from build123d import *

# Parameters (mm, degrees)
BASE_EXTRUDE_DEPTH = 12.7
LPATTERN1_COUNT    = 2
LPATTERN1_PITCH    = 20.6375


with BuildPart() as part:
    # Sketch1 → Base-Extrude (new, symmetric)
    with BuildSketch(Plane.XY):
        with BuildLine():
            Line((-20.6375, 9.37895), (-20.6375, -7.874))
            ThreePointArc((-20.6375, -7.874), (-20.33992049, -8.59242049), (-19.6215, -8.89))
            Line((-19.6215, -8.89), (-1.016, -8.89))
            ThreePointArc((-1.016, -8.89), (-0.29757951, -8.59242049), (0, -7.874))
            Line((0, -7.874), (0, 9.37895))
            ThreePointArc((0, 9.37895), (-2.38125, 11.7602), (-4.7625, 9.37895))
            Line((-4.7625, 9.37895), (-3.7465, 9.37895))
            ThreePointArc((-3.7465, 9.37895), (-2.38125, 10.7442), (-1.016, 9.37895))
            Line((-1.016, 9.37895), (-1.016, -7.874))
            Line((-1.016, -7.874), (-19.6215, -7.874))
            Line((-19.6215, -7.874), (-19.6215, 9.37895))
            ThreePointArc((-19.6215, 9.37895), (-18.25625, 10.7442), (-16.891, 9.37895))
            Line((-16.891, 9.37895), (-15.875, 9.37895))
            ThreePointArc((-15.875, 9.37895), (-18.25625, 11.7602), (-20.6375, 9.37895))
        make_face()
    base_extrude = extrude(amount=BASE_EXTRUDE_DEPTH, both=True)

    # LPattern1: Base-Extrude ×2
    with Locations(*[(i * LPATTERN1_PITCH, 0, 0) for i in range(1, LPATTERN1_COUNT)]):
        add(base_extrude)


solid = part.part
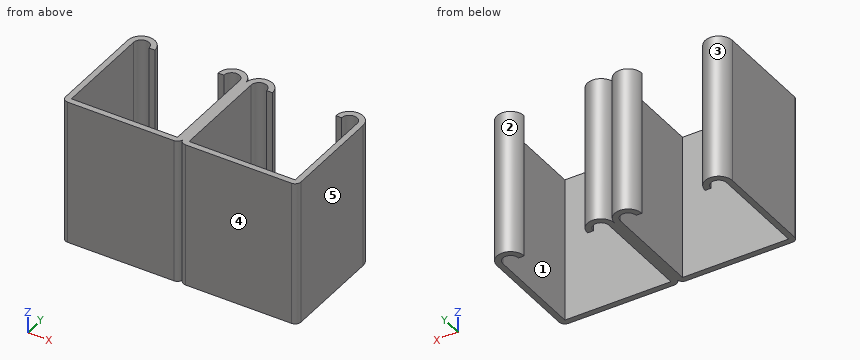
Read the model definition and answer for the solid it produces. Units are mm, in the model's axes. Face numbers are marked on the shaded views. A direction names the side the tool comes from. Give positions to 0.01 mm unless a question says otherwise; leave off trailing zeros. Write each loop counter-clockwise with the first axis right and the second up, starting at its lowest first coordinate (ties: lowest second). Pieces come first, ordered by that corner, then holes. Notation, with made-up numbers: (-37, 23.5) - (1, 23.5) arc R9 ccw to (1, 33.5) - close; hole circle Ø6 at (83.5, 81.5). An arc over 180 degrees is marked (long way). Use CSV: the item, a comma, the result in double quotes. Start each with the question number.
Item 1: The part is cut by section D-D, the plane x = 14. Give the vertices of the cut face in (y, z), and give its area (3 significant figures).
Item 2: The part is cut by section A-A, the plane y = 6.25. Give the vertices of the cut face in (x, z).
Item 3: The mould has two halves that part along X. Classify the marked faces 3, 4 and 5: pulls with the +X half, pulls with the -X half, needs draft (parallel to the pull), parting line crosses it, or undercut.
Item 4: The part is cut by section B-B, the plane x = -1.5. Give the vertices of the cut face in (y, z).
Item 5: Flat-ended cylindrical pins translate along their axes: P1, Ø5, axis at x = -9, y = 9.5, coming from the -Z side; P2, Ø9.5, axis at x = -9, z = -2, coming from the +Y side. Find the tip coordinate at first contact, or state that the pin passes through.
Item 6: Consider line 1 (X direction, y = 4.5, z = 5); line 2 (Y direction, x = -10, z = -3.5); line 3 (Y direction, x = 18.5, z = 9.75). Determine where each line is inside the solid, lowest interval first.
Item 7: The part is cut by section C-C, the plane z = -1.5. Give the vertices of the cut face in (x, y) (1 decimal), and give its area (3 significant figures).
Item 8: For the marked faces 1 and 2, determine the directions among +Z, -Z, +X, -X, +Y, -Y from which every point of the face is accessible in a straight line to the end or side of a thin tool.
Taken from the geometry:
1,outline,"(-8.89, -12.7) - (-7.87, -12.7) - (-7.87, 12.7) - (-8.89, 12.7) - close"
1,area,"25.8 mm2"
2,outline,"(-20.64, -12.7) - (-19.62, -12.7) - (-19.62, 12.7) - (-20.64, 12.7) - close; (-1.02, -12.7) - (1.02, -12.7) - (1.02, 12.7) - (-1.02, 12.7) - close; (19.62, -12.7) - (20.64, -12.7) - (20.64, 12.7) - (19.62, 12.7) - close"
3,face 3,"undercut"
3,face 4,"needs draft"
3,face 5,"pulls with the +X half"
4,outline,"(-8.89, -12.7) - (-7.87, -12.7) - (-7.87, 12.7) - (-8.89, 12.7) - close; (10.42, -12.7) - (11.59, -12.7) - (11.59, 12.7) - (10.42, 12.7) - close"
5,P1,"through"
5,P2,"y = 10.85"
6,line 1,"-20.64 to -19.62, -1.02 to 1.02, 19.62 to 20.64"
6,line 2,"-8.89 to -7.87"
6,line 3,"-8.89 to -7.87, 10.72 to 11.75"
7,outline,"(-20.6, -7.9) arc R1 ccw to (-19.6, -8.9) - (-1, -8.9) arc R1 ccw to (0, -7.9) arc R1 ccw to (1, -8.9) - (19.6, -8.9) arc R1 ccw to (20.6, -7.9) - (20.6, 9.4) arc R2.4 ccw to (15.9, 9.4) - (16.9, 9.4) arc R1.4 cw to (19.6, 9.4) - (19.6, -7.9) - (1, -7.9) - (1, 9.4) arc R1.4 cw to (3.7, 9.4) - (4.8, 9.4) arc R2.4 ccw to (0, 9.4) arc R2.4 ccw to (-4.8, 9.4) - (-3.7, 9.4) arc R1.4 cw to (-1, 9.4) - (-1, -7.9) - (-19.6, -7.9) - (-19.6, 9.4) arc R1.4 cw to (-16.9, 9.4) - (-15.9, 9.4) arc R2.4 ccw to (-20.6, 9.4) - close"
7,area,"135 mm2"
8,face 1,"+Z, -Z"
8,face 2,"+Z, -Z, +Y"
